from build123d import *

# Parameters (mm, degrees)
F1_DEPTH  = 14.5
F2_R      = 3.15
F3_DEPTH  = 14.5
F4_SIZE   = 0.2
F5_W      = 3.287728643
F5_H      = 0.8
F5_W_2    = 2.4924869649
F6_DEPTH  = 14.5
F8_DEPTH  = 85
F9_R      = 16.1404886934
F9_R_2    = 5.65
F10_DEPTH = 10
F10_TAPER = 9.9
F11_R     = 17.5534972963
F11_R_2   = 5.65
F12_DEPTH = 25
F12_TAPER = 10
F14_DEPTH = 10
F16_DEPTH = 10


with BuildPart() as f1:
    # F0 (on Top) → F1 (new body)
    with BuildSketch(Plane.XY):
        Polygon((-3.45, -4.4), (0, -4.4), (3.45, -4.4), (6.9, -0.95), (6.9, 0.95), (3.45, 4.4), (-3.45, 4.4), (-6.9, 0.95), (-6.9, -0.95), align=None)
    extrude(amount=F1_DEPTH)

    # F2 (on face) → F3 (join)
    with BuildSketch(Plane.XY.offset(14.5)):
        Circle(F2_R)
    extrude(amount=F3_DEPTH)

    # F4
    f4_edges = [f1.edges().sort_by_distance(p)[0] for p in [
        (-3.15, 0, 29),
    ]]
    chamfer(f4_edges, length=F4_SIZE)

    # F5 (on face) → F6 (cut)
    with BuildSketch(Plane.XY.offset(29)):
        with Locations((1.6438643215, -2.75)):
            Rectangle(F5_W, F5_H)
        with Locations((-1.2462434825, -2.75)):
            Rectangle(F5_W_2, F5_H)
    extrude(amount=-F6_DEPTH, mode=Mode.SUBTRACT)

    # F7 (on face) → F8 (join)
    with BuildSketch(Plane(origin=(0, 0, 0), x_dir=(1, 0, 0), z_dir=(0, 0, -1))):
        Polygon((3.6373066959, -6.3), (7.2746133918, 0), (3.6373066959, 6.3), (-3.6373066959, 6.3), (-7.2746133918, 0), (-3.6373066959, -6.3), align=None)
    extrude(amount=F8_DEPTH)

    # F9 (on face) → F10 (cut)
    with BuildSketch(Plane.XY):
        Circle(F9_R)
        Circle(F9_R_2, mode=Mode.SUBTRACT)
    extrude(amount=-F10_DEPTH, taper=F10_TAPER, mode=Mode.SUBTRACT)

    # F11 (on face) → F12 (cut)
    with BuildSketch(Plane(origin=(0, 0, -85), x_dir=(1, 0, 0), z_dir=(0, 0, -1))):
        Circle(F11_R)
        Circle(F11_R_2, mode=Mode.SUBTRACT)
    extrude(amount=-F12_DEPTH, taper=F12_TAPER, mode=Mode.SUBTRACT)

    # F13 (on face) → F14 (join)
    with BuildSketch(Plane(origin=(0, 0, -85), x_dir=(1, 0, 0), z_dir=(0, 0, -1))):
        Polygon((-4, -5.5), (0, -5.5), (4, -5.5), (8, -1.5), (8, 0), (8, 1.5), (4, 5.5), (0, 5.5), (-4, 5.5), (-8, 1.5), (-8, 0), (-8, -1.5), align=None)
    extrude(amount=F14_DEPTH)

    # F15 (on face) → F16 (join)
    with BuildSketch(Plane(origin=(0, 0, -95), x_dir=(1, 0, 0), z_dir=(0, 0, -1))):
        Polygon((-3.7, -4.9), (0, -4.9), (3.7, -4.9), (7.4, -1.2), (7.4, 0), (7.4, 1.2), (3.7, 4.9), (0, 4.9), (-3.7, 4.9), (-7.4, 1.2), (-7.4, 0), (-7.4, -1.2), align=None)
    extrude(amount=F16_DEPTH)


solid = f1.part
The listing builds one solid part. Answer for the finished solid, in the listing's coordinates (mm). A direction names the side the tool comes from. Give positions to 0.01 mm unless a question says otherwise; leave off trailing zeros. Order: outer loops, then holes, each group sorted by start corner. A loop starts at its lowest first (then second) coordinate and runs counter-clockwise, first axis right, second up. Notation, with made-up numbers: (-32.5, 30.25) - (10.5, 30.25) arc R18 cw to (10.5, 34.25) - close; hole circle Ø5 at (69.25, 30). An arc over 180 degrees is marked (long way). One line per item, written item: value. Start each with the question number.
1) Find the intervals of material crossed by L1, parallel to Y at x = 2.25, z = 4.5; L2, parallel to Z at x = 3.75, y = -0.5; L3, parallel to X at y = 0, z = -59, in increasing order.
2) Given pin 1 Ø0.7 at (x, y) = (2, 4) entering from +Z; pin 2 Ø0.6 at (y, z) = (0, 5) entering from -X; pin 3 Ø6.5 at (x, z) = (-1.5, -91) entering from -Y; pin 4 Ø7.5 at (x, y) = (5, 1.5) entering from +Z, each flat-ended and moving along its own axis, determine where each tip first touches the part or whether it passes through.
3) A tool of negligible diameter and unlimited length cuts with its end or side. For faces 1 (the face through (0, 4.9, -100)), 2 (the face through (-5.2, -2.65, 7.15)), 3 (the face through (-5.5, -3.1, -99.9)), 4 (the face through (0, -3, 14.5)), from which of +Z, -Z, +X, -X, +Y, -Y can it reach the whole face along a straight path? Write none if from no direction.
4) The mould has two halves that part along Z. Classify faces 5 (the face through (-7.4, 0, -100)), 6 (the face through (6, 0, 0)), 7 (the face through (0, 0, 29)): released by +Z, released by -Z, zero draft, split by the parting line, or undercut.
5) A cutting plane is placed at A-A on x = 0. Give the vertices of the cut face in (y, z), then the cut area to 3 significant figures.
6) A cutting plane is placed at B-B on z = -52. Give the vertices of the cut face in (x, y).
7) A cutting plane is placed at C-C on z = -83. Give the vertices of the cut face in (x, y).
Answer sheet:
1. L1: y = -4.4 to 4.4
1. L2: z = -105 to 14.5
1. L3: x = -7.27 to 7.27
2. pin 1: stops at z = 14.5
2. pin 2: stops at x = -6.9
2. pin 3: stops at y = -5.5
2. pin 4: stops at z = 29
3. face 1: -Z, +X, -X, +Y
3. face 2: +Z, -X, -Y
3. face 3: -Z, -X, -Y
3. face 4: +Z
4. face 5: zero draft
4. face 6: undercut
4. face 7: released by +Z
5. outline: (-6.3, -81.31) - (-5.65, -85) - (-5.5, -85) - (-5.5, -95) - (-4.9, -95) - (-4.9, -105) - (4.9, -105) - (4.9, -95) - (5.5, -95) - (5.5, -85) - (5.65, -85) - (6.3, -81.31) - (6.3, -3.72) - (5.65, 0) - (4.4, 0) - (4.4, 14.5) - (3.15, 14.5) - (3.15, 28.8) - (2.95, 29) - (-2.35, 29) - (-2.35, 14.5) - (-4.4, 14.5) - (-4.4, 0) - (-5.65, 0) - (-6.3, -3.72) - close
5. area: 1,480 mm2
6. outline: (-7.27, 0) - (-3.64, -6.3) - (3.64, -6.3) - (7.27, 0) - (3.64, 6.3) - (-3.64, 6.3) - close
7. outline: circle Ø12.01 at (0, 0)
